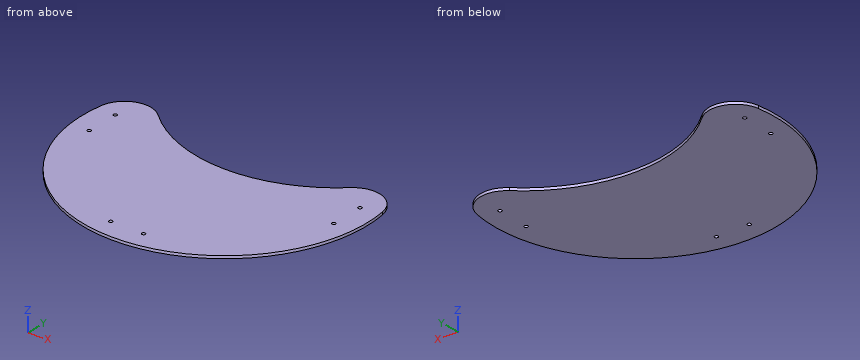
from build123d import *

# Parameters (mm, degrees)
SKETCH_1_R      = 2
EXTRUDE_1_DEPTH = 3


with BuildPart() as part:
    # 草图1 → 凸台-拉伸1 (new body)
    with BuildSketch(Plane.XY):
        with BuildLine():
            ThreePointArc((-158.095170199, 24.615384615), (0, -160), (158.095170199, 24.615384615))
            ThreePointArc((158.095170199, 24.615384615), (138.371023625, 48.312884579), (108.17037961, 42.105263158))
            ThreePointArc((108.17037961, 42.105263158), (0, 0), (-108.17037961, 42.105263158))
            ThreePointArc((-108.17037961, 42.105263158), (-138.371023625, 48.312884579), (-158.095170199, 24.615384615))
        make_face()
        with Locations((137.799674336, 18.195823561)):
            Circle(SKETCH_1_R, mode=Mode.SUBTRACT)
        with Locations((137.799674336, -18.804176439)):
            Circle(SKETCH_1_R, mode=Mode.SUBTRACT)
        with Locations((18.195823561, -137.799674336)):
            Circle(SKETCH_1_R, mode=Mode.SUBTRACT)
        with Locations((-18.804176439, -137.799674336)):
            Circle(SKETCH_1_R, mode=Mode.SUBTRACT)
        with Locations((-137.799674336, -18.195823561)):
            Circle(SKETCH_1_R, mode=Mode.SUBTRACT)
        with Locations((-137.799674336, 18.804176439)):
            Circle(SKETCH_1_R, mode=Mode.SUBTRACT)
    extrude(amount=EXTRUDE_1_DEPTH)


solid = part.part
Work out the finished part from the listing and answer in its coordinate system (mm). Round coordinates to 2 decimals unless told otherwise and drop trailing zeros. Order: outer loops, then holes, each group sorted by start corner. A loop starts at its lowest first (then second) coordinate and runs counter-clockwise, first axis right, second up. Notation, with made-up numbers: M -6,13.25 L 15,13.25 A20 cw 15,40.25 Z; hole C 23,31.25 d6. An arc over 180 degrees is marked long. Put each result on its own line as item: value. Start each with the question number.
Q1. Section C-C, the plane y = -145.5 is taken. Write down the section's boundary in (x, z), and give its area (3 significant figures).
Q2. Section B-B, the plane x = -90 is taken. Write down the section's boundary in (y, z), and give its area (3 significant figures).
Q3. Section A-A, the plane z = 2.3 is taken. Write down the section's boundary in (x, y).
Q4. Straight lines are drawn through the part: L1, parallel to Y at x = 139, z = 1; L2, parallel to X at y = 19, z = 0.25; L3, parallel to X at y = 41.5, z = 1.05. For each, find the intervals that lie inside material, in ascending order. Write a range as [from, to].
Findings below:
1. outline: M -66.56,0 L 66.56,0 L 66.56,3 L -66.56,3 Z
1. area: 399 mm^2
2. outline: M -132.29,0 L 27.71,0 L 27.71,3 L -132.29,3 Z
2. area: 480 mm^2
3. outline: M -158.1,24.62 A160 ccw long 158.1,24.62 A30 ccw 108.17,42.11 A160 cw -108.17,42.11 A30 ccw Z; hole C -137.8,-18.2 d4; hole C -137.8,18.8 d4; hole C -18.8,-137.8 d4; hole C 18.2,-137.8 d4; hole C 137.8,-18.8 d4; hole C 137.8,18.2 d4
4. L1: y = [-79.24, -20.4], [-17.2, 16.6], [19.8, 48.08]
4. L2: x = [-158.87, -139.79], [-135.81, -75.62], [75.62, 135.97], [139.63, 158.87]
4. L3: x = [-149.37, -107.51], [107.51, 149.37]
